Here's how the part is built. I have some questions about the finished solid (model axes, mm). Round coordinates to 2 decimals unless told otherwise and drop trailing zeros. Write each loop counter-clockwise with the first axis right and the second up, starting at its lowest first coordinate (ties: lowest second). Pieces come first, ordered by that corner, then holes. Notation, with made-up numbers: (51, 31.25) - (84, 31.25) arc R9 cw to (84, 46.25) - close; hole circle Ø2 at (46.5, 25). An arc over 180 degrees is marked (long way). Return JSON: item names as keys, results as strings. Group by question number.
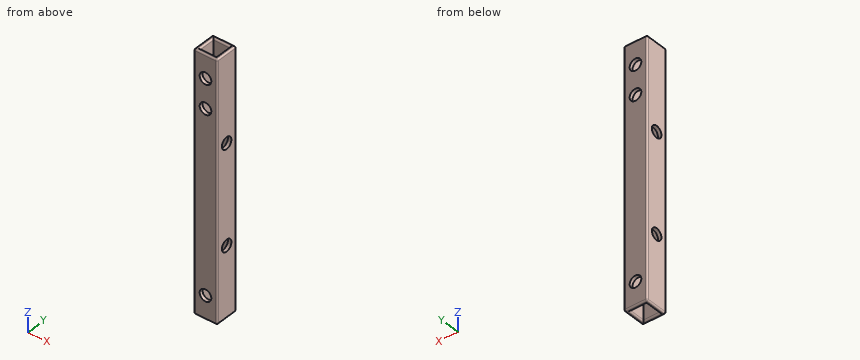
Autodesk Inventor part; units mm, degrees
ref_plane "YZ Plane" through (0, 0, 0) normal (1, 0, 0) x (0, 1, 0)
ref_plane "XZ Plane" through (0, 0, 0) normal (0, 1, 0) x (-1, 0, 0)
ref_plane "XY Plane" through (0, 0, 0) normal (0, 0, 1) x (1, 0, 0)
sketch "Sketch1" plane through (0, 0, 0) normal (0, 0, 1) x (1, 0, 0)
  line L0 (0, 0) -> (25.4, 0)
  line L1 (25.4, 0) -> (25.4, 25.4)
  line L2 (25.4, 25.4) -> (0, 25.4)
  line L3 (0, 25.4) -> (0, 0)
  dimension "d0" = 25.4
  dimension "d1" = 25.4
extrude "Extrusion1" add sketch "Sketch1" along normal blind 279.4
sketch "Sketch2" plane through (0, 25.4, 0) normal (0, 1, 0) x (1, 0, 0)
  line L0 (0, 0) -> (0, -279.4)
  line L1 (25.4, 0) -> (25.4, -279.4)
  line L2 (0, 0) -> (0, -25.4)
  line L3 (0, -25.4) -> (12.7, -25.4)
  circle A0 centre (12.7, -25.4) radius 6.35
  line L4 (25.4, -279.4) -> (25.4, -254)
  line L5 (25.4, -254) -> (12.7, -254)
  circle A1 centre (12.7, -254) radius 6.35
  dimension "d4" = 25.4
  dimension "d5" = 12.7
  dimension "d6" = 25.4
  dimension "d7" = 12.7
extrude "Extrusion2" cut sketch "Sketch2" against normal blind 279.4
sketch "Sketch3" plane through (0, 0, 0) normal (0, 0, -1) x (-1, 0, 0)
  line L0 (0, 0) -> (-25.4, 0)
  line L1 (-25.4, 25.4) -> (0, 25.4)
  line L2 (-25.4, 0) -> (-25.4, 25.4)
  line L3 (-25.4, 25.4) -> (-25.4, 21.59)
  line L4 (-25.4, 21.59) -> (-21.59, 21.59)
  line L5 (-25.4, 0) -> (-21.59, 0)
  line L6 (-21.59, 0) -> (-21.59, 3.81)
  line L7 (0, 0) -> (-3.81, 0)
  line L8 (-3.81, 0) -> (-3.81, 3.81)
  line L9 (0, 25.4) -> (-3.81, 25.4)
  line L10 (-3.81, 25.4) -> (-3.81, 21.59)
  line L11 (-3.81, 21.59) -> (-21.59, 21.59)
  line L12 (-21.59, 21.59) -> (-21.59, 3.81)
  line L13 (-21.59, 3.81) -> (-3.81, 3.81)
  line L14 (-3.81, 3.81) -> (-3.81, 21.59)
  dimension "d10" = 3.81
  dimension "d11" = 3.81
  dimension "d12" = 3.81
  dimension "d13" = 3.81
  dimension "d14" = 3.81
  dimension "d15" = 3.81
  dimension "d16" = 3.81
  dimension "d17" = 3.81
extrude "Extrusion3" cut sketch "Sketch3" against normal blind 279.4 contours L13 L12 L11 L14
sketch "Sketch4" plane through (0, 0, 0) normal (0, -1, 0) x (1, 0, 0)
  circle A0 centre (12.7, 254) radius 6.35
  line L0 (0, 0) -> (0, 279.4)
  line L1 (12.7, 247.65) -> (12.7, 222.25)
  circle A1 centre (12.7, 222.25) radius 6.35
  dimension "d20" = 25.4
  dimension "d21" = 12.7
extrude "Extrusion4" cut sketch "Sketch4" against normal blind 279.4 contours A1
sketch "Sketch5" plane through (0, 25.4, 0) normal (0, 1, 0) x (1, 0, 0)
  circle A0 centre (12.7, -222.25) radius 6.35
  circle A1 centre (12.7, -25.4) radius 6.35
  circle A2 centre (12.7, -254) radius 6.35
  line L0 (25.4, 0) -> (0, 0)
  line L1 (0, 0) -> (0, -279.4)
  line L2 (25.4, -279.4) -> (0, -279.4)
  line L3 (25.4, 0) -> (25.4, -279.4)
sketch "Sketch6" plane through (25.4, 0, 0) normal (1, 0, 0) x (0, 0, -1)
  line L0 (0, 25.4) -> (-279.4, 25.4)
  line L1 (0, 0) -> (-279.4, 0)
  line L2 (-222.6507, 25.4) -> (-222.6507, 12.7)
  line L3 (-222.6507, 12.7) -> (-184.5507, 12.7)
  circle A0 centre (-184.5507, 12.7) radius 6.35
  line L4 (-178.2007, 12.7) -> (-76.6007, 12.7)
  circle A1 centre (-76.6007, 12.7) radius 6.35
  dimension "d25" = 12.7
  dimension "d24" = 38.1
  dimension "d26" = 101.6
  dimension "d27" = 12.7
extrude "Extrusion5" cut sketch "Sketch6" against normal blind 279.4
fillet "Fillet1" radius 1.5875 20 edges at (0, 0, 139.7) (0, 25.4, 139.7) (12.7, 25.4, 279.4) (12.7, 0, 279.4) (25.4, 12.7, 279.4) (0, 12.7, 279.4) (25.4, 25.4, 139.7) (25.4, 0, 139.7) (25.4, 12.7, 0) (12.7, 25.4, 0) (12.7, 21.59, 0) (3.81, 12.7, 0) (0, 12.7, 0) (12.7, 0, 0) (12.7, 3.81, 0) (21.59, 12.7, 0) (3.81, 12.7, 279.4) (12.7, 21.59, 279.4) (21.59, 12.7, 279.4) (12.7, 3.81, 279.4)
properties part number "Vertical Rod" material "Steel"
1) Imagine slicing it at A-A (y = 12.7). Give the number of separate pieces and of enclosed holes in the cut face, plus the area to 3 significant figures.
2) I need wall thicknesses on line 1 along Y through (x, z) = (8, 140); line 2 along Z through (x, y) = (12.7, 22.8). Which ranges of each line are inside material? Lowest first, please.
3) Imagine slicing it at C-C (z = 61). Please give me the cut outline in (x, y) (1 decimal).
Results found:
{
 "1": {"separate pieces": "6", "enclosed holes": "0", "area": "1,930 mm²"},
 "2": {"line 1": "y = 0 to 3.81, 21.59 to 25.4", "line 2": "z = 0.05 to 19.05, 31.75 to 215.9, 228.6 to 247.65, 260.35 to 279.35"},
 "3": {"outline": "(0, 1.6) arc R1.6 ccw to (1.6, 0) - (23.8, 0) arc R1.6 ccw to (25.4, 1.6) - (25.4, 23.8) arc R1.6 ccw to (23.8, 25.4) - (1.6, 25.4) arc R1.6 ccw to (0, 23.8) - close; hole (3.8, 3.8) - (21.6, 3.8) - (21.6, 21.6) - (3.8, 21.6) - close"}
}
